from build123d import *

# Parameters (mm, degrees)
SKETCH_R        = 2
SKETCH_W        = 110.5
SKETCH_H        = 54
PAD_DEPTH       = 6
SKETCH001_W     = 16
SKETCH001_H     = 6
PAD001_DEPTH    = 14
SKETCH002_R     = 2
HOLE_DEPTH      = 24
SKETCH003_R     = 3
POCKET_DEPTH    = 2
CHAMFER_SIZE    = 1
CHAMFER001_SIZE = 1
FILLET_R        = 3
CHAMFER002_SIZE = 10


with BuildPart() as part:
    # Sketch → Pad (new body)
    with BuildSketch(Plane.XY):
        Polygon((143, -7), (0.5, -7), (0.5, 108), (16.5, 108), (16.5, 61), (127, 61), (127, 108), (143, 108), align=None)
        with Locations((8.5, 15)):
            Circle(SKETCH_R, mode=Mode.SUBTRACT)
        with Locations((8.5, 100)):
            Circle(SKETCH_R, mode=Mode.SUBTRACT)
        with Locations((135, 15)):
            Circle(SKETCH_R, mode=Mode.SUBTRACT)
        with Locations((135, 100)):
            Circle(SKETCH_R, mode=Mode.SUBTRACT)
        with Locations((71.75, 26)):
            Rectangle(SKETCH_W, SKETCH_H, mode=Mode.SUBTRACT)
    extrude(amount=PAD_DEPTH)

    # Sketch001 (on Face18 of Pad) → Pad001 (join)
    with BuildSketch(Plane.XY.offset(6)):
        with Locations((135, -4)):
            Rectangle(SKETCH001_W, SKETCH001_H)
        with Locations((8.5, -4)):
            Rectangle(SKETCH001_W, SKETCH001_H)
    extrude(amount=PAD001_DEPTH)

    # Sketch002 (on DatumPlane) → Hole (cut)
    with BuildSketch(Plane(origin=(0, -1, 0), x_dir=(-1, 0, 0), z_dir=(0, 1, 0))):
        with Locations((-135, 12)):
            Circle(SKETCH002_R)
        with Locations((-8.5, 12)):
            Circle(SKETCH002_R)
    extrude(amount=-HOLE_DEPTH, mode=Mode.SUBTRACT)

    # Sketch003 (on Face20 of Hole) → Pocket (cut)
    with BuildSketch(Plane(origin=(0, -1, 0), x_dir=(-1, 0, 0), z_dir=(0, 1, 0))):
        with Locations((-135, 12)):
            Circle(SKETCH003_R)
        with Locations((-8.5, 12)):
            Circle(SKETCH003_R)
    extrude(amount=-POCKET_DEPTH, mode=Mode.SUBTRACT)

    # Chamfer
    chamfer_edges = [part.edges().sort_by_distance(p)[0] for p in [
        (6.5, 15, 0),
        (6.5, 100, 0),
        (133, 15, 0),
        (133, 100, 0),
    ]]
    chamfer(chamfer_edges, length=CHAMFER_SIZE)

    # Chamfer001
    chamfer001_edges = [part.edges().sort_by_distance(p)[0] for p in [
        (11.5, -1, 12),
        (138, -1, 12),
    ]]
    chamfer(chamfer001_edges, length=CHAMFER001_SIZE)

    # Fillet
    fillet_edges = [part.edges().sort_by_distance(p)[0] for p in [
        (0.5, 108, 3),
        (16.5, 108, 3),
        (127, 108, 3),
        (143, 108, 3),
        (0.5, -4, 20),
        (16.5, -4, 20),
        (127, -4, 20),
        (143, -4, 20),
    ]]
    fillet(fillet_edges, radius=FILLET_R)

    # Chamfer002
    chamfer002_edges = [part.edges().sort_by_distance(p)[0] for p in [
        (16.5, 61, 3),
        (16.5, 53, 3),
        (127, 61, 3),
        (127, 53, 3),
    ]]
    chamfer(chamfer002_edges, length=CHAMFER002_SIZE)


solid = part.part
Design review of the part built by this model. Coordinates are the model's own, in mm. A direction names the side the tool comes from. Coordinates: 2 decimals unless noted, no trailing zeros. Order: outer loops, then holes, each group sorted by start corner. A loop starts at its lowest first (then second) coordinate and runs counter-clockwise, first axis right, second up.
Item 1: For faces 1 (the flat face through (72, 58, 6)), 2 (the cylindrical face through (15.64, -3.96, 19.1)), 3 (the cylindrical face through (132.14, -2.49, 12.9)), list the 3-axis set-ups (+Z, -Z, +X, -X, +Y, -Y) from which the entire face can be reached by the end or side of a thin tool; tool diameter is ignored.
Item 2: The part is to be moulded in two halves that separate along Z. For faces 4 (the cylindrical face through (8.76, -4.972, 13.983)), 5 (the flat face through (122, 48, 3)), 6 (the cylindrical face through (5.73, -2.49, 10.85)), 7 (the flat face through (8, -4, 20)), say which applies: pulls with the +Z half, pulls with the -Z half, needs draft (parallel to the pull), parting line crosses it, or undercut.
Item 3: Take a section at C-C, the plane y = 51. Write out the cut boundary in (x, z).
Item 4: Take a section at A-A, the plane z = 12. Write out the cut boundary in (x, y), then the cut area to 3 significant figures.
Item 5: For line 1 (Y direction, x = 135, z = 2.7); line 2 (Y direction, x = 133.5, z = 2.5); line 3 (Z direction, x = 8.5, y = -2.4), list the stretches that pass through material, from the lowest coordinate up.
Item 6: Take a section at D-D, the plane x = 135. Write out the cut boundary in (y, z), then the cut area to 3 significant figures.
Item 7: Take a section at B-B, the plane x = 95. Write out the cut boundary in (y, z).
Item 8: For pin 1 Ø5 at (x, z) = (135, 12) entering from +Y; pin 2 Ø6 at (x, z) = (60, 6) entering from +Y; pin 3 Ø4.5 at (x, y) = (135, 100) entering from +Z, all flat-tipped, find the tip position at first contact; note any pin that passes through.
The answers:
1. face 1: +Z, +X, -X, +Y
1. face 2: +Z, +Y, -Y
1. face 3: +Y
2. face 4: undercut
2. face 5: needs draft
2. face 6: undercut
2. face 7: pulls with the +Z half
3. outline: (0.5, 0) - (24.5, 0) - (24.5, 6) - (0.5, 6) - close; (119, 0) - (143, 0) - (143, 6) - (119, 6) - close
4. outline: (0.5, -7) - (6.5, -7) - (6.5, -3) - (5.5, -3) - (5.5, -2) - (4.5, -1) - (0.5, -1) - close; (10.5, -7) - (16.5, -7) - (16.5, -1) - (12.5, -1) - (11.5, -2) - (11.5, -3) - (10.5, -3) - close; (127, -7) - (133, -7) - (133, -3) - (132, -3) - (132, -2) - (131, -1) - (127, -1) - close; (137, -7) - (143, -7) - (143, -1) - (139, -1) - (138, -2) - (138, -3) - (137, -3) - close
4. area: 134 mm2
5. line 1: y = -7 to 13, 17 to 98, 102 to 108
5. line 2: y = -7 to 13.68, 16.32 to 98.68, 101.32 to 108
5. line 3: z = 0 to 9, 15 to 20
6. outline: (-7, 0) - (12, 0) - (13, 1) - (13, 6) - (-1, 6) - (-1, 8) - (-2, 9) - (-3, 9) - (-3, 10) - (-7, 10) - close; (-7, 14) - (-3, 14) - (-3, 15) - (-2, 15) - (-1, 16) - (-1, 20) - (-7, 20) - close; (17, 1) - (18, 0) - (97, 0) - (98, 1) - (98, 6) - (17, 6) - close; (102, 1) - (103, 0) - (108, 0) - (108, 6) - (102, 6) - close
6. area: 695 mm2
7. outline: (-7, 0) - (-1, 0) - (-1, 6) - (-7, 6) - close; (53, 0) - (61, 0) - (61, 6) - (53, 6) - close
8. pin 1: stops at y = -3
8. pin 2: stops at y = 61
8. pin 3: stops at z = 6
